```python
from build123d import *

# Parameters (mm, degrees)
F0_R     = 2.4892
F0_R_2   = 14.29512
F1_DEPTH = 3.81
F2_DEPTH = 9.525
F3_DEPTH = 3.81
F4_R     = 1.27
F5_R     = 1.27


with BuildPart() as f1:
    # F0 (on Front) → F1 (new body)
    with BuildSketch(Plane.XZ):
        with BuildLine():
            Line((22.068503, 28.572265), (-23.40348, 28.572265))
            ThreePointArc((-23.40348, 28.572265), (-24.801539, 28.41645), (-26.130988, 27.956652))
            Line((-26.130988, 27.956652), (-26.130988, -27.950701))
            ThreePointArc((-26.130988, -27.950701), (-24.790565, -28.418992), (-23.379597, -28.577735))
            Line((-23.379597, -28.577735), (22.04462, -28.577735))
            ThreePointArc((22.04462, -28.577735), (23.455588, -28.418992), (24.796012, -27.950701))
            Line((24.796012, -27.950701), (24.796012, 27.956652))
            ThreePointArc((24.796012, 27.956652), (23.466562, 28.41645), (22.068503, 28.572265))
        make_face()
        with Locations((-12.573738, -20.624965)):
            Circle(F0_R, mode=Mode.SUBTRACT)
        with Locations((-21.289718, -11.908985)):
            Circle(F0_R, mode=Mode.SUBTRACT)
        with Locations((-0.667488, -23.815235)):
            Circle(F0_R, mode=Mode.SUBTRACT)
        with Locations((11.238762, -20.624965)):
            Circle(F0_R, mode=Mode.SUBTRACT)
        with Locations((-0.667488, -0.002735)):
            Circle(F0_R_2, mode=Mode.SUBTRACT)
        with Locations((19.954742, -11.908985)):
            Circle(F0_R, mode=Mode.SUBTRACT)
        with Locations((-21.289718, 11.903515)):
            Circle(F0_R, mode=Mode.SUBTRACT)
        with Locations((-12.573738, 20.619495)):
            Circle(F0_R, mode=Mode.SUBTRACT)
        with Locations((-0.667488, 23.809765)):
            Circle(F0_R, mode=Mode.SUBTRACT)
        with Locations((19.954742, 11.903515)):
            Circle(F0_R, mode=Mode.SUBTRACT)
        with Locations((11.238762, 20.619495)):
            Circle(F0_R, mode=Mode.SUBTRACT)
        with Locations((-0.667488, -0.002735)):
            Circle(F0_R_2)
        Polygon((-8.014501, -0.002735), (-4.340995, 6.359965), (3.006018, 6.359965), (6.679525, -0.002735), (3.006018, -6.365435), (-4.340995, -6.365435), align=None, mode=Mode.SUBTRACT)
        with BuildLine():
            ThreePointArc((26.599113, 26.671543), (25.754008, 27.393295), (24.796012, 27.956652))
            Line((24.796012, 27.956652), (24.796012, -27.950701))
            ThreePointArc((24.796012, -27.950701), (25.757368, -27.379239), (26.603558, -26.647982))
            Line((26.603558, -26.647982), (31.09275, -22.017935))
            ThreePointArc((31.09275, -22.017935), (32.137376, -20.198047), (32.186375, -18.100229))
            Line((32.186375, -18.100229), (29.346901, -5.723291))
            ThreePointArc((29.346901, -5.723291), (28.703786, -0.003786), (29.364856, 5.713672))
            Line((29.364856, 5.713672), (32.240124, 18.068518))
            ThreePointArc((32.240124, 18.068518), (32.191617, 20.214999), (31.115326, 22.072774))
            Line((31.115326, 22.072774), (26.599113, 26.671543))
        make_face()
        with Locations((28.034512, -19.052735)):
            Circle(F0_R, mode=Mode.SUBTRACT)
        with Locations((28.034512, 19.047265)):
            Circle(F0_R, mode=Mode.SUBTRACT)
        with BuildLine():
            Line((-26.130988, -27.950701), (-26.130988, 27.956652))
            ThreePointArc((-26.130988, 27.956652), (-27.088985, 27.393295), (-27.934089, 26.671543))
            Line((-27.934089, 26.671543), (-32.450303, 22.072774))
            ThreePointArc((-32.450303, 22.072774), (-33.526593, 20.214999), (-33.575101, 18.068518))
            Line((-33.575101, 18.068518), (-30.699833, 5.713672))
            ThreePointArc((-30.699833, 5.713672), (-30.038763, -0.003786), (-30.681878, -5.723291))
            Line((-30.681878, -5.723291), (-33.521351, -18.100229))
            ThreePointArc((-33.521351, -18.100229), (-33.472352, -20.198047), (-32.427726, -22.017935))
            Line((-32.427726, -22.017935), (-27.938535, -26.647982))
            ThreePointArc((-27.938535, -26.647982), (-27.092345, -27.379239), (-26.130988, -27.950701))
        make_face()
        with Locations((-29.369488, -19.052735)):
            Circle(F0_R, mode=Mode.SUBTRACT)
        with Locations((-29.369488, 19.047265)):
            Circle(F0_R, mode=Mode.SUBTRACT)
    extrude(amount=F1_DEPTH)

    # F0 (on Front) → F2 (join)
    with BuildSketch(Plane.XZ):
        with Locations((-0.667488, -0.002735)):
            Circle(F0_R_2)
        Polygon((-8.014501, -0.002735), (-4.340995, 6.359965), (3.006018, 6.359965), (6.679525, -0.002735), (3.006018, -6.365435), (-4.340995, -6.365435), align=None, mode=Mode.SUBTRACT)
    extrude(amount=F2_DEPTH)

    # F0 (on Front) → F3 (join)
    with BuildSketch(Plane.XZ):
        with BuildLine():
            Line((-26.130988, -27.950701), (-26.130988, 27.956652))
            ThreePointArc((-26.130988, 27.956652), (-27.088985, 27.393295), (-27.934089, 26.671543))
            Line((-27.934089, 26.671543), (-32.450303, 22.072774))
            ThreePointArc((-32.450303, 22.072774), (-33.526593, 20.214999), (-33.575101, 18.068518))
            Line((-33.575101, 18.068518), (-30.699833, 5.713672))
            ThreePointArc((-30.699833, 5.713672), (-30.038763, -0.003786), (-30.681878, -5.723291))
            Line((-30.681878, -5.723291), (-33.521351, -18.100229))
            ThreePointArc((-33.521351, -18.100229), (-33.472352, -20.198047), (-32.427726, -22.017935))
            Line((-32.427726, -22.017935), (-27.938535, -26.647982))
            ThreePointArc((-27.938535, -26.647982), (-27.092345, -27.379239), (-26.130988, -27.950701))
        make_face()
        with Locations((-29.369488, -19.052735)):
            Circle(F0_R, mode=Mode.SUBTRACT)
        with Locations((-29.369488, 19.047265)):
            Circle(F0_R, mode=Mode.SUBTRACT)
        with BuildLine():
            ThreePointArc((26.599113, 26.671543), (25.754008, 27.393295), (24.796012, 27.956652))
            Line((24.796012, 27.956652), (24.796012, -27.950701))
            ThreePointArc((24.796012, -27.950701), (25.757368, -27.379239), (26.603558, -26.647982))
            Line((26.603558, -26.647982), (31.09275, -22.017935))
            ThreePointArc((31.09275, -22.017935), (32.137376, -20.198047), (32.186375, -18.100229))
            Line((32.186375, -18.100229), (29.346901, -5.723291))
            ThreePointArc((29.346901, -5.723291), (28.703786, -0.003786), (29.364856, 5.713672))
            Line((29.364856, 5.713672), (32.240124, 18.068518))
            ThreePointArc((32.240124, 18.068518), (32.191617, 20.214999), (31.115326, 22.072774))
            Line((31.115326, 22.072774), (26.599113, 26.671543))
        make_face()
        with Locations((28.034512, -19.052735)):
            Circle(F0_R, mode=Mode.SUBTRACT)
        with Locations((28.034512, 19.047265)):
            Circle(F0_R, mode=Mode.SUBTRACT)
    extrude(amount=-F3_DEPTH)

    # F4
    f4_edges = [f1.edges().sort_by_distance(p)[0] for p in [
        (-14.962608, -9.525, -0.002735),
    ]]
    fillet(f4_edges, radius=F4_R)

    # F5
    f5_edges = [f1.edges().sort_by_distance(p)[0] for p in [
        (-14.962608, -3.81, -0.002735),
    ]]
    fillet(f5_edges, radius=F5_R)


solid = f1.part
```
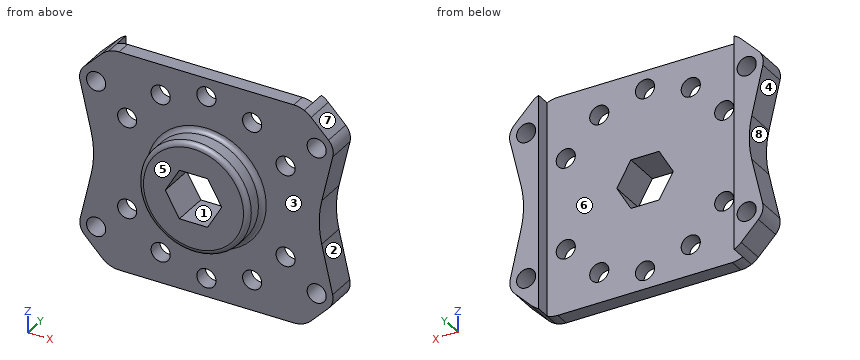
Geometry check sheet. Reference: the model listing, model coordinates, mm. Face numbers are marked on the shaded views. A direction names the side the tool comes from. Round coordinates to 2 decimals unless told otherwise and drop trailing zeros. Loops run counter-clockwise (first coordinate to the right, second up) from the corner with the lowest first, then second, coordinate; pieces in that order, holes last. Notation, with made-up numbers: (54.5, 17.25) - (67.5, 17.25) arc R26 cw to (67.5, 31.25) - close; hole circle Ø8 at (79.25, 60.5). An arc over 180 degrees is marked (long way). Use a Markdown table: item, result.
Q1. Go/stop test with flat-tipped pins: P1, Ø5.5, axis at x = -29.37, z = 19.05, coming from the +Y side; P2, Ø6.5, axis at x = 19.95, z = 11.9, coming from the -Y side; P3, Ø1.9, axis at y = 1.5, z = -13, coming from the +X side; P4, Ø4, axis at y = -8, z = -9, coming from the +X side. Record where each tip stops, or that it passes through.
Solutions:
| item | result |
|---|---|
| P1 | stops at y = 3.81 |
| P2 | stops at y = -3.81 |
| P3 | stops at x = 31.23 |
| P4 | stops at x = 11.8 |
Q2. Cross-section at C-C on x = -11. State how many separate pieces and enclosed holes the cut face has, plus the area to 3 significant figures.
Solutions:
| item | result |
|---|---|
| separate pieces | 3 |
| enclosed holes | 0 |
| area | 301 mm2 |
Q3. Draft check along Z on the marked faces 6, 7 and 8. Enter one of: released by +Z, released by -Z, zero draft, split by the parting line, or undercut.
Solutions:
| item | result |
|---|---|
| face 6 | zero draft |
| face 7 | released by +Z |
| face 8 | undercut |
Q4. Material ranges on line 1 (X direction, y = -1.75, z = -22); line 2 (X direction, y = -0.5, z = -18); line 3 (X direction, y = -1, z = 11.5), recorded low to high.
Solutions:
| item | result |
|---|---|
| line 1 | x = -32.45 to -14.65, -10.5 to -2.37, 1.04 to 9.16, 13.31 to 31.11 |
| line 2 | x = -33.5 to -31.63, -27.11 to 25.78, 30.29 to 32.16 |
| line 3 | x = -32.05 to -23.75, -18.83 to 17.5, 22.41 to 30.71 |
Q5. Cross-section at B-B on y = 0.75. Record the cut outline in (x, z), plus the area to 3 significant figures.
Solutions:
| item | result |
|---|---|
| outline | (-33.58, 18.07) - (-30.7, 5.71) arc R25.4 cw to (-30.68, -5.72) - (-33.52, -18.1) arc R4.26 ccw to (-32.43, -22.02) - (-27.94, -26.65) arc R6.35 ccw to (-26.13, -27.95) - (-26.13, 27.96) arc R6.35 ccw to (-27.93, 26.67) - (-32.45, 22.07) arc R4.32 ccw to start; (24.8, -27.95) arc R6.35 ccw to (26.6, -26.65) - (31.09, -22.02) arc R4.26 ccw to (32.19, -18.1) - (29.35, -5.72) arc R25.4 cw to (29.36, 5.71) - (32.24, 18.07) arc R4.32 ccw to (31.12, 22.07) - (26.6, 26.67) arc R6.35 ccw to (24.8, 27.96) - close; hole circle Ø4.98 at (-29.37, -19.05); hole circle Ø4.98 at (-29.37, 19.05); hole circle Ø4.98 at (28.03, -19.05); hole circle Ø4.98 at (28.03, 19.05) |
| area | 507 mm2 |
Q6. Access from +Z, -Z, +X, -X, +Y, -Y to the whole of each face (thin tool, end or side, straight path). Record for the marked faces 1, 2, 3, 4 and 5.
Solutions:
| item | result |
|---|---|
| face 1 | +Y, -Y |
| face 2 | +X, +Y, -Y |
| face 3 | -Y |
| face 4 | -X, +Y, -Y |
| face 5 | +Z, -Z, +X, -X, -Y |
Q7. Cross-section at A-A on x = 20. Record the cut outline in (y, z).
Solutions:
| item | result |
|---|---|
| outline | (-3.81, -28.58) - (0, -28.58) - (0, -14.4) - (-3.81, -14.4) - close; (-3.81, -9.42) - (0, -9.42) - (0, 9.41) - (-3.81, 9.41) - close; (-3.81, 14.39) - (0, 14.39) - (0, 28.57) - (-3.81, 28.57) - close |
